Autodesk Inventor part; units mm, degrees
ref_plane "YZ Plane" through (0, 0, 0) normal (1, 0, 0) x (0, 1, 0)
ref_plane "XZ Plane" through (0, 0, 0) normal (0, 1, 0) x (-1, 0, 0)
ref_plane "XY Plane" through (0, 0, 0) normal (0, 0, 1) x (1, 0, 0)
sketch "スケッチ1" plane through (0, 0, 0) normal (0, 1, 0) x (-1, 0, 0)
  line L0 (0, 0) -> (7.8, 0)
  line L1 (7.8, 0) -> (7.8, -20)
  line L2 (7.8, -20) -> (0, -20)
  line L3 (0, -20) -> (0, 0)
  line L4 (0, -5.5) -> (3.3, -5.5)
  line L5 (3.3, -5.5) -> (3.3, -14.5)
  line L6 (3.3, -14.5) -> (0, -14.5)
  line L7 (0, -14.5) -> (0, -5.5)
  dimension "d0" = 7.8
  dimension "d1" = 20
  dimension "d2" = 3.3
  dimension "d3" = 9
  dimension "d4" = 5.5
extrude "押し出し1" add sketch "スケッチ1" along normal blind 30 contours L0 L1 L2 L3 L6 L5 L4
sketch "スケッチ2" plane through (-7.8, 0, -20) normal (-1, 0, 0) x (0, 0, 1)
  line L0 (17.5, 30.0313) -> (17.5, 0)
  line L1 (2.5, 30.0313) -> (2.5, 0)
  line L2 (20, 0) -> (20, 30)
  line L3 (0, 0) -> (0, 30)
  line L4 (0, 30) -> (20, 30)
  point P0 (2.5, 20)
  point P1 (2.5, 10)
  point P2 (17.5, 20)
  point P3 (17.5, 10)
  dimension "d7" = 2.5
  dimension "d8" = 2.5
  dimension "d9" = 10
  dimension "d10" = 10
  dimension "d11" = 10
  dimension "d12" = 10
hole "穴1" at (-7.8, 20, -17.5) at (-7.8, 10, -17.5) at (-7.8, 20, -2.5) at (-7.8, 10, -2.5) direction (1, 0, 0) diameter 3 depth 3 tip angle 118
properties part number "linear_SSEB10"
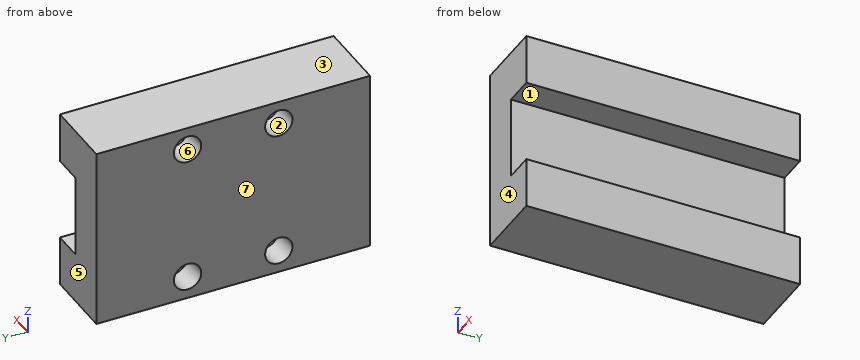
Source: CAD feature listing. Evaluate the final solid. Frame: model axes, mm. Face numbers are marked on the shaded views. A direction names the side the tool comes from. Coordinates: 2 decimals unless noted, no trailing zeros. Loops run counter-clockwise (first coordinate to the right, second up) from the corner with the lowest first, then second, coordinate; pieces in that order, holes last. Notation, with made-up numbers: M 17.5,80 L 25.5,80 A15 cw 25.5,85 Z; hole C -17.75,34 d11. An arc over 180 degrees is marked long. Answer in a Markdown table with one row per item.
Q1. Section D-D on z = -8.5. Return the cut outline in (x, y).
Answers below:
| item | result |
|---|---|
| outline | M -7.8,0 L -3.3,0 L -3.3,30 L -7.8,30 Z |
Q2. Section A-A on x = -1. Return the cut outline in (y, z), plus the area to 3 significant figures.
Answers below:
| item | result |
|---|---|
| outline | M 0,-20 L 30,-20 L 30,-14.5 L 0,-14.5 Z; M 0,-5.5 L 30,-5.5 L 30,0 L 0,0 Z |
| area | 330 mm^2 |
Q3. Section B-B on y = 3.25. Return the cut outline in (x, z).
Answers below:
| item | result |
|---|---|
| outline | M -7.8,-20 L 0,-20 L 0,-14.5 L -3.3,-14.5 L -3.3,-5.5 L 0,-5.5 L 0,0 L -7.8,0 Z |
Q4. First-contact query: pin 1 (2.5 mm diameter, centred on y = 20, z = -17.5, fed in from -X); pin 2 (7 mm diameter, centred on y = 20.5, z = -10, fed in from +X). Flat tips, straight axial feed; report the tip coordinate or a pass-through.
Answers below:
| item | result |
|---|---|
| pin 1 | stops at x = -4.65 |
| pin 2 | stops at x = -3.3 |
Q5. Section C-C on x = -6.75. Return the cut outline in (y, z), plus the area to 3 significant figures.
Answers below:
| item | result |
|---|---|
| outline | M 0,-20 L 30,-20 L 30,0 L 0,0 Z; hole C 10,-17.5 d3; hole C 10,-2.5 d3; hole C 20,-17.5 d3; hole C 20,-2.5 d3 |
| area | 572 mm^2 |
Q6. Set-up query: the marked faces 1, 2 and 3. Return all of +Z, -Z, +X, -X, +Y, -Y with unobstructed straight access to the full face (end or side cutting, diameter ignored); none if empty.
Answers below:
| item | result |
|---|---|
| face 1 | +X, +Y, -Y |
| face 2 | -X |
| face 3 | +Z, +X, -X, +Y, -Y |
Q7. Ray query, probe 1 along Z at (x, y) = (-6.4, 20); probe 2 along Y at (x, z) = (-5.9, -17.5); probe 3 along Z at (x, y) = (-3, 18.25). Return the intervals inside material, ascending. Write a range as from..to.
Answers below:
| item | result |
|---|---|
| probe 1 | z = -20..-19, -16..-4, -1..0 |
| probe 2 | y = 0..8.5, 11.5..18.5, 21.5..30 |
| probe 3 | z = -20..-14.5, -5.5..0 |
Q8. Draft query along Y for the marked faces 4, 5, 6 and 7. Return one class per face: pulls with the +Y half, pulls with the -Y half, needs draft (parallel to the pull), parting line crosses it, or undercut.
Answers below:
| item | result |
|---|---|
| face 4 | pulls with the -Y half |
| face 5 | pulls with the +Y half |
| face 6 | undercut |
| face 7 | needs draft |
